```python
from build123d import *

# Parameters (mm, degrees)
SKETCH1_R           = 5.175
BOSS_EXTRUDE1_DEPTH = 2.5


with BuildPart() as part:
    # Sketch1 → Boss-Extrude1 (new body)
    with BuildSketch(Plane(origin=(0, 0, 0), x_dir=(1, 0, 0), z_dir=(0, 1, 0))):
        Polygon((0, 8.25), (-7.144709581, 4.125), (-7.144709581, -4.125), (0, -8.25), (7.144709581, -4.125), (7.144709581, 4.125), align=None)
        with Locations(Location((0, 0, 0), (0, 0, 270))):
            Circle(SKETCH1_R, mode=Mode.SUBTRACT)
    extrude(amount=BOSS_EXTRUDE1_DEPTH)

    # Sketch2 → Cut-Revolve3 (revolve, cut)
    with BuildSketch(Plane(origin=(1.914419162, 0, 0), x_dir=(1, 0, 0), z_dir=(0, 0, 1)), mode=Mode.PRIVATE) as cut_revolve3_sk:
        with BuildLine():
            Line((-1.914419162, 3.174819063), (-1.914419162, 16.07690266))
            ThreePointArc((-1.914419162, 16.07690266), (-17.205966927, 0.785354895), (-1.914419162, -14.506192869))
            Line((-1.914419162, -14.506192869), (-1.914419162, -0.674819063))
            ThreePointArc((-1.914419162, -0.674819063), (-7.281350854, -0.189682365), (-12.47429107, 1.25))
            ThreePointArc((-12.47429107, 1.25), (-7.281350854, 2.689682365), (-1.914419162, 3.174819063))
        make_face()
    revolve(cut_revolve3_sk.sketch.rotate(Axis((0, 4.297603661, 0), (0, -1, 0)), 270), axis=Axis((0, 4.297603661, 0), (0, -1, 0)), mode=Mode.SUBTRACT)


solid = part.part
```
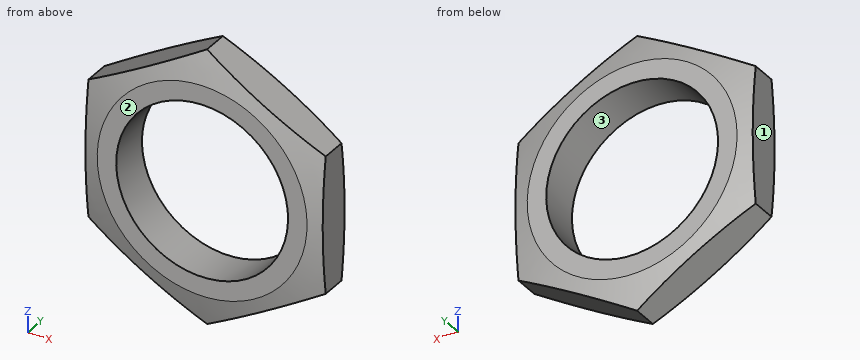
Verification items for the finished model (mm, model axes). Face numbers are marked on the shaded views. Give positions to 0.01 mm unless a question says otherwise; leave off trailing zeros. Order: outer loops, then holes, each group sorted by start corner. A loop starts at its lowest first (then second) coordinate and runs counter-clockwise, first axis right, second up. Notation, with made-up numbers: (53.5, 50) -> (99.5, 50) arc R10 cw to (99.5, 67) -> close; hole circle Ø8 at (38, -38). An arc over 180 degrees is marked (long way). Use a Markdown table: item, result.
1) Section check A-A, the plane z = 0. Record the boundary of the cut face in (x, y) (3 decimals).
Results:
| item | result |
|---|---|
| outline | (-7.145, 0.19) arc R29.929 ccw to (-6.32, 0) -> (-5.175, 0) -> (-5.175, 2.5) -> (-6.32, 2.5) arc R29.929 ccw to (-7.145, 2.31) -> close; (5.175, 0) -> (6.32, 0) arc R29.929 ccw to (7.145, 0.19) -> (7.145, 2.31) arc R29.929 ccw to (6.32, 2.5) -> (5.175, 2.5) -> close |
2) Section check B-B, the plane y = 0.75. Record the boundary of the cut face in (x, z) (3 decimals).
Results:
| item | result |
|---|---|
| outline | (-7.145, -4.125) -> (0, -8.25) -> (7.145, -4.125) -> (7.145, 4.125) -> (0, 8.25) -> (-7.145, 4.125) -> close; hole circle Ø10.35 at (0, 0) |
3) Section check D-D, the plane x = -5.5. Record the boundary of the cut face in (y, z).
Results:
| item | result |
|---|---|
| outline | (0, -3.11) arc R29.42 ccw to (0.28, -5.07) -> (2.22, -5.07) arc R29.42 ccw to (2.5, -3.11) -> (2.5, 3.11) arc R29.42 ccw to (2.22, 5.07) -> (0.28, 5.07) arc R29.42 ccw to (0, 3.11) -> close |
4) Section check C-C, the plane x = 4.5. Record the boundary of the cut face in (y, z), then the cut area to 3 significant figures.
Results:
| item | result |
|---|---|
| outline | (0, -4.44) arc R29.59 ccw to (0.21, -5.65) -> (2.29, -5.65) arc R29.59 ccw to (2.5, -4.44) -> (2.5, -2.56) -> (0, -2.56) -> close; (0, 2.56) -> (2.5, 2.56) -> (2.5, 4.44) arc R29.59 ccw to (2.29, 5.65) -> (0.21, 5.65) arc R29.59 ccw to (0, 4.44) -> close |
| area | 15.0 mm² |
5) Mould release check, pull along X, two halves, no side actions. Record for the marked faces 1, 2 and 3: pulls with the +X half, pulls with the -X half, needs draft (parallel to the pull), parting line crosses it, or undercut.
Results:
| item | result |
|---|---|
| face 1 | pulls with the -X half |
| face 2 | needs draft |
| face 3 | undercut |
6) Material ranges on probe 1 along X at (y, z) = (0.9, 0) (3 decimals); probe 2 along X at (y, z) = (1.15, -1); probe 3 along Z at (x, y) = (1, 1.95), recorded low to high.
Results:
| item | result |
|---|---|
| probe 1 | -7.145 to -5.175, 5.175 to 7.145 |
| probe 2 | -7.14 to -5.08, 5.08 to 7.14 |
| probe 3 | -7.67 to -5.08, 5.08 to 7.67 |
